Geometry: see drawing. Coordinates: mm, zero at the bounding-box minimum. A direction names the side the tool comes from. Give positions to 0.01 mm unless a question says otherwise; leave off trailing zeros. Order: outer loops, then holes, each group sorted by start corner. A loop starts at its lowest first (then second) coordinate and runs counter-clockwise, first axis right, second up. Notation, with made-up numbers: (-30, 43) - (18, 43) arc R25 ccw to (18, 69) - close; hole circle Ø11 at (64, 38). An arc over 180 degrees is marked (long way). Write each question's results on one line, items separated by ' | '. Start each with the question number.
Item 1: Set-up query: the marked faces 5 and 6. Return all of +Z, -Z, +X, -X, +Y, -Y with unobstructed straight access to the full face (end or side cutting, diameter ignored); none if empty.
Item 2: Mould query, pull axis X, two halves, no side actions, for the marked faces 1, 2, 3 and 4. Classes: released by +X, released by -X, zero draft, split by the parting line, or undercut.
Item 3: Line query: line 1 along X through (y, z) = (20.75, 9.75); line 2 along Z through (x, y) = (4.5, 23.5); line 3 along X through (y, z) = (10.75, 23). Output: solid intervals per line, ascending.
Item 4: Section A-A on z = 16.25. Output: boundary loops of the cut face in (x, y).
Item 5: Contact query for a flat-ended pin moving along its axis: pin 1 Ø12 at (x, z) = (38.5, 3) entering from +Y. Output: stop coordinate, or through.
Item 6: Section C-C on x = 38.5. Output: boundary loops of the cut face in (y, z), and give its area (3 significant figures).
Item 7: Section B-B on y = 5.5. Output: boundary loops of the cut face in (x, z).
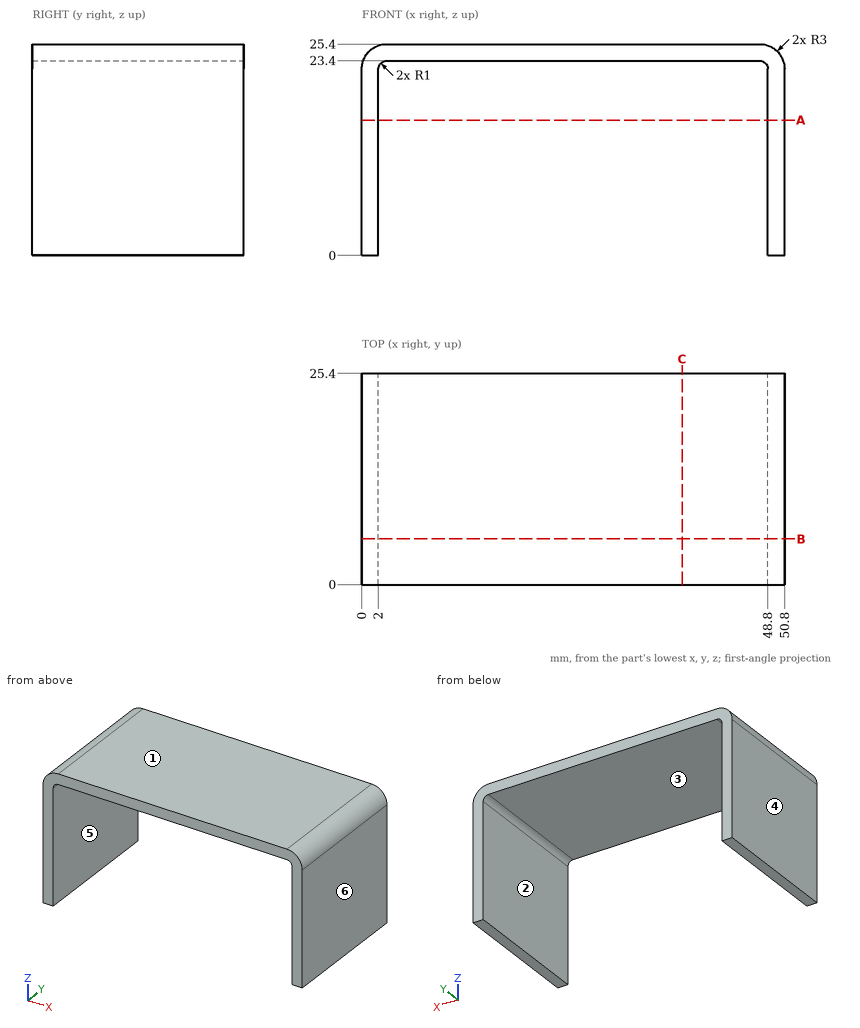
Evaluation:
1) face 5: -Z, +Y, -Y | face 6: +Z, -Z, +X, +Y, -Y
2) face 1: zero draft | face 2: undercut | face 3: undercut | face 4: released by -X
3) line 1: x = 0 to 2, 48.8 to 50.8 | line 2: z = 23.4 to 25.4 | line 3: x = 0.06 to 2.2, 48.6 to 50.74
4) outline: (0, 0) - (2, 0) - (2, 25.4) - (0, 25.4) - close; (48.8, 0) - (50.8, 0) - (50.8, 25.4) - (48.8, 25.4) - close
5) pin 1: passes through
6) outline: (0, 23.4) - (25.4, 23.4) - (25.4, 25.4) - (0, 25.4) - close | area: 50.8 mm^2
7) outline: (0, 0) - (2, 0) - (2, 22.4) arc R1 cw to (3, 23.4) - (47.8, 23.4) arc R1 cw to (48.8, 22.4) - (48.8, 0) - (50.8, 0) - (50.8, 22.4) arc R3 ccw to (47.8, 25.4) - (3, 25.4) arc R3 ccw to (0, 22.4) - close
